Model file for the job. Use its own axes, mm. A direction names the side the tool comes from. Coordinates: 2 decimals unless noted, no trailing zeros. Write each loop counter-clockwise with the first axis right and the second up, starting at its lowest first coordinate (ties: lowest second). Pieces come first, ordered by that corner, then holes.
Q1. Pull direction Y, two halves, no side cores. Call faces 1 (the flat face through (39, 16.603, 2)), 2 (the cylindrical face through (1.66, 20.5, 1.57)), 3 (the flat face through (39, 19.143, 2)): released by +Y, released by -Y, zero draft, split by the parting line, or undercut.
Q2. Band-saw the part on B-B, the plane z = 0.55. Write the cut outline in (x, y), plus the area to 3 significant figures.
Q3. Drill centre lines: probe 1 along X at (y, z) = (20.25, 0.3); probe 2 along Y at (x, z) = (52, 2.1); probe 3 along X at (y, z) = (19.25, 2.7). Where is each one in solid material? Low to high.
Q4. Which spindle directions (+Z, -Z, +X, -X, +Y, -Y) get a long thin tool onto all of the face, cutting with end or side? Do faces 4 (the cylindrical face through (64.742, 20.385, 1.565)), 5 (the flat face through (40, 24.223, 2)). Say none if no direction does.
Q5. Band-saw the part on A-A, the plane x = 16.5. Write the cut outline in (y, z) (3 decimals), plus the area to 3 significant figures.
Q6. Band-saw the part on C-C, the plane y = 19.75. State how many separate pieces and enclosed holes the cut face has, plus the area to 3 significant figures.
from build123d import *

# Parameters (mm, degrees)
BOSS_EXTRUDE1_DEPTH                               = 3.175
CSK_FOR_4_FLAT_HEAD_MACHINE_SCREW_100_D           = 3.4544
CSK_FOR_4_FLAT_HEAD_MACHINE_SCREW_100_CSINK_D     = 6.925818
CSK_FOR_4_FLAT_HEAD_MACHINE_SCREW_100_CSINK_ANGLE = 100
CUT_EXTRUDE1_DEPTH                                = 4.175


with BuildPart() as part:
    # Sketch1 → Boss-Extrude1 (new body)
    with BuildSketch(Plane.XY):
        with BuildLine():
            Line((5.469571116, 16.602717302), (72.76915781, 16.602717302))
            ThreePointArc((72.76915781, 16.602717302), (76.57915781, 20.412717302), (72.76915781, 24.222717302))
            Line((72.76915781, 24.222717302), (5.469571116, 24.222717302))
            ThreePointArc((5.469571116, 24.222717302), (1.659571116, 20.412717302), (5.469571116, 16.602717302))
        make_face()
    extrude(amount=BOSS_EXTRUDE1_DEPTH)

    # CSK for #4 Flat Head Machine Screw (100)1 (through all)
    with Locations(Plane.XY.offset(3.175)):
        with Locations((5.469571116, 20.412717302), (72.76915781, 20.412717302)):
            CounterSinkHole(CSK_FOR_4_FLAT_HEAD_MACHINE_SCREW_100_D / 2, CSK_FOR_4_FLAT_HEAD_MACHINE_SCREW_100_CSINK_D / 2, counter_sink_angle=CSK_FOR_4_FLAT_HEAD_MACHINE_SCREW_100_CSINK_ANGLE)

    # Sketch4 → Cut-Extrude1 (cut, through all)
    with BuildSketch(Plane(origin=(0, 0, 0), x_dir=(-1, 0, 0), z_dir=(0, 0, -1))):
        with BuildLine():
            Line((-63.47275781, 21.682717302), (-14.765971116, 21.682717302))
            ThreePointArc((-14.765971116, 21.682717302), (-13.495971116, 20.412717302), (-14.765971116, 19.142717302))
            Line((-14.765971116, 19.142717302), (-63.47275781, 19.142717302))
            ThreePointArc((-63.47275781, 19.142717302), (-64.74275781, 20.412717302), (-63.47275781, 21.682717302))
        make_face()
    extrude(amount=-CUT_EXTRUDE1_DEPTH, mode=Mode.SUBTRACT)


solid = part.part
Answer sheet:
1. face 1: released by -Y
1. face 2: split by the parting line
1. face 3: undercut
2. outline: (5.47, 16.6) - (72.77, 16.6) arc R3.81 ccw to (72.77, 24.22) - (5.47, 24.22) arc R3.81 ccw to start; hole circle Ø3.45 at (5.47, 20.41); hole (14.77, 19.14) - (63.47, 19.14) arc R1.27 ccw to (63.47, 21.68) - (14.77, 21.68) arc R1.27 ccw to start; hole circle Ø3.45 at (72.77, 20.41)
2. area: 411 mm2
3. probe 1: x = 1.66 to 3.75, 7.19 to 13.51, 64.73 to 71.05, 74.49 to 76.58
3. probe 2: y = 16.6 to 19.14, 21.68 to 24.22
3. probe 3: x = 1.84 to 2.82, 8.12 to 14.26, 63.98 to 70.12, 75.42 to 76.4
4. face 4: +Z, -Z
4. face 5: +Z, -Z, +X, -X, +Y
5. outline: (16.603, 0) - (19.143, 0) - (19.143, 3.175) - (16.603, 3.175) - close; (21.683, 0) - (24.223, 0) - (24.223, 3.175) - (21.683, 3.175) - close
5. area: 16.1 mm2
6. separate pieces: 4
6. enclosed holes: 0
6. area: 50.4 mm2
